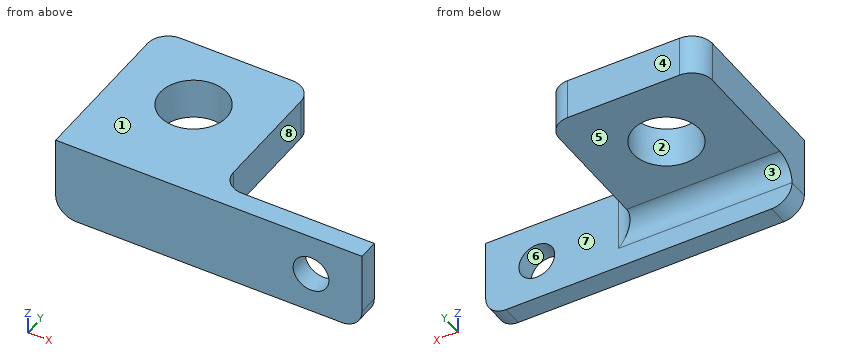
from build123d import *

# Parameters (mm, degrees)
CROQUIS1_W              = 30
CROQUIS1_H              = 8
CROQUIS1_R              = 1.75
SALIENTE_EXTRUIR1_DEPTH = 2
CROQUIS2_W              = 15
CROQUIS2_H              = 4
SALIENTE_EXTRUIR2_DEPTH = 15
CROQUIS3_R              = 3.25
CORTAR_EXTRUIR1_DEPTH   = 4
REDONDEO1_R             = 2


with BuildPart() as part:
    # Croquis1 → Saliente-Extruir1 (new body)
    with BuildSketch(Plane(origin=(0, 0, 0), x_dir=(1, 0, 0), z_dir=(0, 1, 0))):
        with Locations((-15, 4)):
            Rectangle(CROQUIS1_W, CROQUIS1_H)
        with Locations(Location((-5, 4, 0), (0, 0, 270))):
            Circle(CROQUIS1_R, mode=Mode.SUBTRACT)
    extrude(amount=SALIENTE_EXTRUIR1_DEPTH)

    # Croquis2 → Saliente-Extruir2 (add)
    with BuildSketch(Plane(origin=(0, 2, 0), x_dir=(1, 0, 0), z_dir=(0, 1, 0))):
        with Locations((-22.5, 2)):
            Rectangle(CROQUIS2_W, CROQUIS2_H)
    extrude(amount=SALIENTE_EXTRUIR2_DEPTH)

    # Croquis3 → Cortar-Extruir1 (cut)
    with BuildSketch(Plane(origin=(0, 0, -4), x_dir=(-1, 0, 0), z_dir=(0, 0, -1))):
        with Locations((22.5, 10)):
            Circle(CROQUIS3_R)
    extrude(amount=-CORTAR_EXTRUIR1_DEPTH, mode=Mode.SUBTRACT)

    # Redondeo1
    redondeo1_edges = [part.edges().sort_by_distance(p)[0] for p in [
        (0, 1, -8),
        (-30, 1, -8),
        (-30, 17, -2),
        (-15, 17, -2),
        (-22.5, 2, -4),
        (-15, 2, -2),
    ]]
    fillet(redondeo1_edges, radius=REDONDEO1_R - 0.0001)  # a hair under: the kernel refuses the full size


solid = part.part
Geometry: final body of the model. Coordinates: model frame, mm. Face numbers are marked on the shaded views. A direction names the side the tool comes from. Round coordinates to 2 decimals unless told otherwise and drop trailing zeros. Loops run counter-clockwise (first coordinate to the right, second up) from the corner with the lowest first, then second, coordinate; pieces in that order, holes last. Notation, with made-up numbers: M 11,44 L 50,44 A37 ccw 50,83 Z; hole C -23.5,67.25 d5. An arc over 180 degrees is marked long. One line per question, with ' | ' between items.
(1) Contact query for flat-ended pins moving along their axis: P1, Ø4, axis at x = -25, y = 13.5, coming from the -Z side; P2, Ø3, axis at y = 12, z = -2, coming from the +X side. Output: stop coordinate, or through.
Check result:
P1: stops at z = -4 | P2: stops at x = -15
(2) Pull-direction query (Y, two-part tool) for the marked faces 1, 2 and 3; classes: +Y half, -Y half, draft (parallel to the pull), parting line (faces both ways), or undercut.
Check result:
face 1: draft | face 2: undercut | face 3: +Y half
(3) Material intervals for line 1 along Y through (x, z) = (-22.5, -1.85); line 2 along X through (y, z) = (0.7, -4); line 3 along Y through (x, z) = (-8.5, -3.5), sorted ascending. Write a range as from..to.
Check result:
line 1: y = 0..6.75, 13.25..17 | line 2: x = -30..-6.75, -3.25..0 | line 3: y = 0..2
(4) Cut plane C-C on z = -1.5. Return the cut outline in (x, y).
Check result:
outline: M -30,0 L 0,0 L 0,2 L -13,2 A2 cw -15,4 L -15,15 A2 ccw -17,17 L -28,17 A2 ccw -30,15 Z; hole C -22.5,10 d6.5
(5) Cut plane D-D on z = -5. Return the cut outline in (x, y), plus the area to 3 significant figures.
Check result:
outline: M -30,0 L -6.44,0 L -6.44,2 L -13,2 A2 cw -14,2.27 L -30,2.27 Z; M -3.56,0 L 0,0 L 0,2 L -3.56,2 Z | area: 58.6 mm2
(6) Cut plane B-B on y = 10. Return the cut outline in (x, z).
Check result:
outline: M -30,-4 L -25.75,-4 L -25.75,0 L -30,0 Z; M -19.25,-4 L -15,-4 L -15,0 L -19.25,0 Z
(7) Cut plane A-A on x = -5. Return the cut outline in (y, z).
Check result:
outline: M 0,-8 L 2,-8 L 2,-5.75 L 0,-5.75 Z; M 0,-2.25 L 2,-2.25 L 2,0 L 0,0 Z
(8) Access query for the marked faces 4, 5, 6, 7 and 8. Directions: +Z, -Z, +X, -X, +Y, -Y. A direction counts if a zero-diameter tool reaches every point of the face in a straight line with its end or side. Return the directions, or none.
Check result:
face 4: +Z, -Z, +X, -X, +Y | face 5: -Z, +X, -X, +Y | face 6: +Y, -Y | face 7: -Z, +X, +Y | face 8: +Z, -Z, +X, +Y
